Work out the finished part from the listing and answer in its coordinate system (mm). A direction names the side the tool comes from. Round coordinates to 2 decimals unless told otherwise and drop trailing zeros. Loops run counter-clockwise (first coordinate to the right, second up) from the corner with the lowest first, then second, coordinate; pieces in that order, holes last.
from build123d import *

# Parameters (mm, degrees)
SKETCH1_W           = 92
SKETCH1_H           = 60
BOSS_EXTRUDE1_DEPTH = 3
CUT_EXTRUDE1_DEPTH  = 3


with BuildPart() as part:
    # Sketch1 → Boss-Extrude1 (new body)
    with BuildSketch(Plane.XY):
        Rectangle(SKETCH1_W, SKETCH1_H)
    extrude(amount=BOSS_EXTRUDE1_DEPTH)

    # Sketch2 → Cut-Extrude1 (cut)
    with BuildSketch(Plane.XY.offset(3)):
        with BuildLine():
            Line((-35, 15), (-10, 15))
            ThreePointArc((-10, 15), (-9, 14), (-10, 13))
            Line((-10, 13), (-35, 13))
            ThreePointArc((-35, 13), (-36, 14), (-35, 15))
        make_face()
        with BuildLine():
            Line((-35, -14), (-10, -14))
            ThreePointArc((-10, -14), (-9, -15), (-10, -16))
            Line((-10, -16), (-35, -16))
            ThreePointArc((-35, -16), (-36, -15), (-35, -14))
        make_face()
        with BuildLine():
            Line((35, 13), (10, 13))
            ThreePointArc((10, 13), (9, 14), (10, 15))
            Line((10, 15), (35, 15))
            ThreePointArc((35, 15), (36, 14), (35, 13))
        make_face()
        with BuildLine():
            Line((35, -16), (10, -16))
            ThreePointArc((10, -16), (9, -15), (10, -14))
            Line((10, -14), (35, -14))
            ThreePointArc((35, -14), (36, -15), (35, -16))
        make_face()
    extrude(amount=-CUT_EXTRUDE1_DEPTH, mode=Mode.SUBTRACT)


solid = part.part
Item 1: For faces 5 (the face through (-1, 0, 3)), 6 (the face through (-36, 14, 2)), determine the directions among +Z, -Z, +X, -X, +Y, -Y from which every point of the face is accessible in a straight line to the end or side of a thin tool.
Item 2: Section C-C, the plane z = 2 is taken. Give the vertices of the cut face in (x, y).
Item 3: A straight line is drawn through the part: line 1 (Y direction, x = 19, z = 2.8). Find the intervals that lie inside material, in ascending order.
Item 4: Section B-B, the plane x = -14 is taken. Give the vertices of the cut face in (y, z), plus the area to 3 significant figures.
Item 5: Section A-A, the plane y = -15 is taken. Give the vertices of the cut face in (x, z), plus the area to 3 significant figures.
Item 6: Determine the mould class of faces 1 (the face through (46, 0, 1)), 2 (the face through (-1, 30, 1)), 3 (the face through (-1, -30, 1)), 4 (the face through (22, 15, 2)) for opening direction Y: pulls with the +Y half, pulls with the -Y half, needs draft (parallel to the pull), parting line crosses it, or undercut.
Answer below:
1. face 5: +Z, +X, -X, +Y, -Y
1. face 6: +Z, -Z
2. outline: (-46, -30) - (46, -30) - (46, 30) - (-46, 30) - close; hole (-35, -16) - (-10, -16) arc R1 ccw to (-10, -14) - (-35, -14) arc R1 ccw to start; hole (-35, 13) - (-10, 13) arc R1 ccw to (-10, 15) - (-35, 15) arc R1 ccw to start; hole (10, -16) - (35, -16) arc R1 ccw to (35, -14) - (10, -14) arc R1 ccw to start; hole (10, 13) - (35, 13) arc R1 ccw to (35, 15) - (10, 15) arc R1 ccw to start
3. line 1: y = -30 to -16, -14 to 13, 15 to 30
4. outline: (-30, 0) - (-16, 0) - (-16, 3) - (-30, 3) - close; (-14, 0) - (13, 0) - (13, 3) - (-14, 3) - close; (15, 0) - (30, 0) - (30, 3) - (15, 3) - close
4. area: 168 mm2
5. outline: (-46, 0) - (-36, 0) - (-36, 3) - (-46, 3) - close; (-9, 0) - (9, 0) - (9, 3) - (-9, 3) - close; (36, 0) - (46, 0) - (46, 3) - (36, 3) - close
5. area: 114 mm2
6. face 1: needs draft
6. face 2: pulls with the +Y half
6. face 3: pulls with the -Y half
6. face 4: undercut
